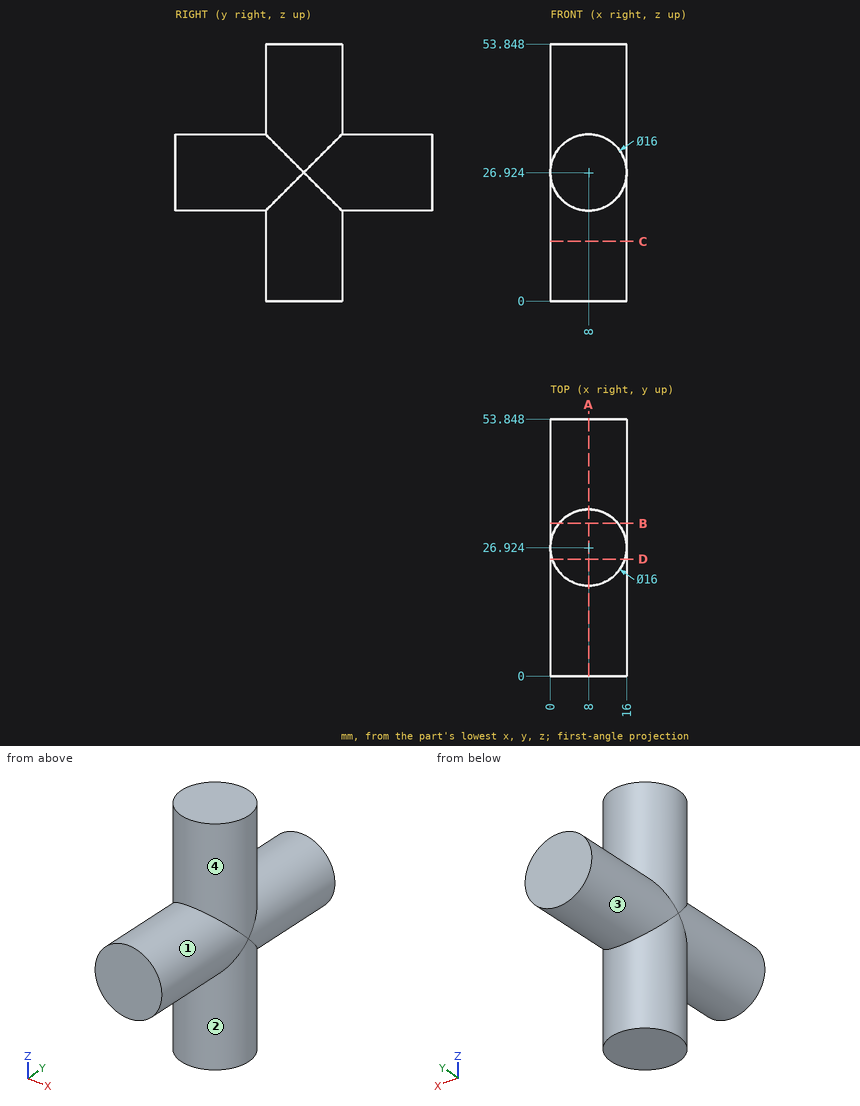
Could you check a few things on this drawing? It's one solid part, dimensions in mm from its lowest x, y, z. A direction names the side the tool comes from. Coordinates: 2 decimals unless noted, no trailing zeros. Loops run counter-clockwise (first coordinate to the right, second up) from the corner with the lowest first, then second, coordinate; pieces in that order, holes last.
1. For the marked faces 1, 2, 3 and 4, which set-ups out of +Z, -Z, +X, -X, +Y, -Y let a thin tool reach every point of the face, with its end or its side?
2. Imagine slicing it at B-B (y = 32). Please give me the cut outline in (x, z).
3. I need wall thicknesses on L1, parallel to X at y = 12.5, z = 26.5; L2, parallel to Y at x = 8.5, z = 43; L3, parallel to Z at x = 3.5, y = 18. Which ranges of each line are inside material? Lowest first, please.
4. Imagine slicing it at C-C (z = 12.5). Please give me the cut outline in (x, y).
5. For P1, Ø2, axis at x = 13, y = 44, coming from the -Z side; P2, Ø1.5, axis at x = 8, z = 6.5, coming from the +Y side; P3, Ø10, axis at y = 17, z = 41.5, coming from the +X side, each with a flat end and sliding along its axis, tell me the tip position at first contact or that it passes through.
6. Imagine slicing it at D-D (y = 24.5). Please give me the cut outline in (x, z).
7. Imagine slicing it at A-A (x = 8). Please give me the cut outline in (y, z).
Computed values:
1. face 1: -Y
1. face 2: -Z
1. face 3: +Y
1. face 4: +Z
2. outline: (1.82, 0) - (14.18, 0) - (14.18, 21.85) arc R8 ccw to (14.18, 32) - (14.18, 53.85) - (1.82, 53.85) - (1.82, 32) arc R8 ccw to (1.82, 21.85) - close
3. L1: x = 0.01 to 15.99
3. L2: y = 18.94 to 34.91
3. L3: z = 20.31 to 33.54
4. outline: circle Ø16 at (8, 26.92)
5. P1: stops at z = 20
5. P2: stops at y = 34.92
5. P3: stops at x = 14.31
6. outline: (0.38, 0) - (15.62, 0) - (15.62, 24.5) arc R8 ccw to (15.62, 29.35) - (15.62, 53.85) - (0.38, 53.85) - (0.38, 29.35) arc R8 ccw to (0.38, 24.5) - close
7. outline: (0, 18.92) - (18.92, 18.92) - (18.92, 0) - (34.92, 0) - (34.92, 18.92) - (53.85, 18.92) - (53.85, 34.92) - (34.92, 34.92) - (34.92, 53.85) - (18.92, 53.85) - (18.92, 34.92) - (0, 34.92) - close
